The model under review builds one solid part; all positions refer to its coordinate system, in mm. Face numbers are marked on the shaded views. A direction names the side the tool comes from. Give positions to 0.01 mm unless a question says otherwise; leave off trailing zeros. Order: outer loops, then holes, each group sorted by start corner. A loop starts at its lowest first (then second) coordinate and runs counter-clockwise, first axis right, second up. Notation, with made-up numbers: (53, -25) - (89, -25) arc R11 ccw to (89, -16) - close; hole circle Ø3 at (-10, 60.5). An arc over 180 degrees is marked (long way). Put each result on its own line as item: value.
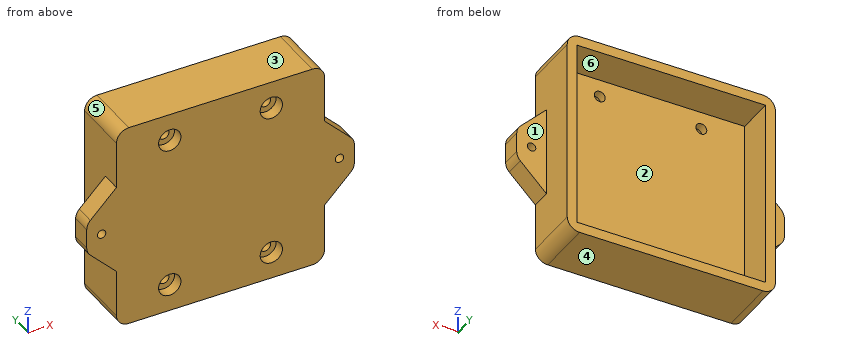
```python
from build123d import *

# Parameters (mm, degrees)
SKETCH1_W           = 84
SKETCH1_H           = 84
SKETCH1_W_2         = 76
SKETCH1_H_2         = 76
SKETCH1_R           = 4.5
SKETCH1_R_2         = 2.2
SKETCH1_W_3         = 12
SKETCH1_H_3         = 12
SKETCH1_R_3         = 1.7
BOSS_EXTRUDE1_DEPTH = 8
SKETCH1_3_W         = 84
SKETCH1_3_H         = 84
SKETCH1_3_W_2       = 76
SKETCH1_3_H_2       = 76
BOSS_EXTRUDE2_DEPTH = 15
SKETCH2_R           = 4.5
CUT_EXTRUDE1_DEPTH  = 4.5
FILLET1_R           = 5


with BuildPart() as part:
    # Sketch1 → Boss-Extrude1 (new body)
    with BuildSketch(Plane(origin=(0, 0, 0), x_dir=(1, 0, 0), z_dir=(0, 1, 0))):
        Rectangle(SKETCH1_W, SKETCH1_H)
        Rectangle(SKETCH1_W_2, SKETCH1_H_2, mode=Mode.SUBTRACT)
        Rectangle(SKETCH1_W_2, SKETCH1_H_2)
        with Locations((20.5, -31)):
            Circle(SKETCH1_R, mode=Mode.SUBTRACT)
        with Locations((-20.5, -31)):
            Circle(SKETCH1_R, mode=Mode.SUBTRACT)
        with Locations((20.5, 31)):
            Circle(SKETCH1_R, mode=Mode.SUBTRACT)
        with Locations((-20.5, 31)):
            Circle(SKETCH1_R, mode=Mode.SUBTRACT)
        with Locations((-20.5, -31)):
            Circle(SKETCH1_R)
        with Locations((-20.5, -31)):
            Circle(SKETCH1_R_2, mode=Mode.SUBTRACT)
        with Locations((-20.5, 31)):
            Circle(SKETCH1_R)
        with Locations((-20.5, 31)):
            Circle(SKETCH1_R_2, mode=Mode.SUBTRACT)
        with Locations((20.5, 31)):
            Circle(SKETCH1_R)
        with Locations((20.5, 31)):
            Circle(SKETCH1_R_2, mode=Mode.SUBTRACT)
        with Locations((20.5, -31)):
            Circle(SKETCH1_R)
        with Locations((20.5, -31)):
            Circle(SKETCH1_R_2, mode=Mode.SUBTRACT)
        Polygon((-42, 6), (-42, 18), (-54, 6), align=None)
        with Locations((-48, 0)):
            Rectangle(SKETCH1_W_3, SKETCH1_H_3)
        with Locations((-48, 0)):
            Circle(SKETCH1_R_3, mode=Mode.SUBTRACT)
        Polygon((-42, -18), (-42, -6), (-54, -6), align=None)
        Polygon((54, 6), (42, 18), (42, 6), align=None)
        with Locations((48, 0)):
            Rectangle(SKETCH1_W_3, SKETCH1_H_3)
        with Locations((48, 0)):
            Circle(SKETCH1_R_3, mode=Mode.SUBTRACT)
        Polygon((54, -6), (42, -6), (42, -18), align=None)
    extrude(amount=-BOSS_EXTRUDE1_DEPTH)

    # Sketch1_3 → Boss-Extrude2 (add)
    with BuildSketch(Plane(origin=(0, 0, 0), x_dir=(1, 0, 0), z_dir=(0, 1, 0))):
        Rectangle(SKETCH1_3_W, SKETCH1_3_H)
        Rectangle(SKETCH1_3_W_2, SKETCH1_3_H_2, mode=Mode.SUBTRACT)
    extrude(amount=BOSS_EXTRUDE2_DEPTH)

    # Sketch2 → Cut-Extrude1 (cut)
    with BuildSketch(Plane.XZ.offset(8)):
        with Locations((-20.5, 31)):
            Circle(SKETCH2_R)
        with Locations((-20.5, -31)):
            Circle(SKETCH2_R)
        with Locations((20.5, -31)):
            Circle(SKETCH2_R)
        with Locations((20.5, 31)):
            Circle(SKETCH2_R)
    extrude(amount=-CUT_EXTRUDE1_DEPTH, mode=Mode.SUBTRACT)

    # Fillet1
    fillet1_edges = [part.edges().sort_by_distance(p)[0] for p in [
        (42, 3.5, 42),
        (-42, 3.5, 42),
        (-54, -4, 6),
        (-54, -4, -6),
        (-42, 3.5, -42),
        (42, 3.5, -42),
        (54, -4, -6),
        (54, -4, 6),
    ]]
    fillet(fillet1_edges, radius=FILLET1_R)


solid = part.part
```
(1) Take a section at C-C, the plane x = -20.5. Write out the cut boundary in (y, z), then the cut area to 3 significant figures.
The answers:
outline: (-8, -42) - (15, -42) - (15, -38) - (0, -38) - (0, -33.2) - (-3.5, -33.2) - (-3.5, -35.5) - (-8, -35.5) - close; (-8, -26.5) - (-3.5, -26.5) - (-3.5, -28.8) - (0, -28.8) - (0, 28.8) - (-3.5, 28.8) - (-3.5, 26.5) - (-8, 26.5) - close; (-8, 35.5) - (-3.5, 35.5) - (-3.5, 33.2) - (0, 33.2) - (0, 38) - (15, 38) - (15, 42) - (-8, 42) - close
area: 680 mm^2
(2) Take a section at D-D, the plane y = 7.25. Write out the cut boundary in (x, z), then the cut area to 3 significant figures.
The answers:
outline: (-42, -37) arc R5 ccw to (-37, -42) - (37, -42) arc R5 ccw to (42, -37) - (42, 37) arc R5 ccw to (37, 42) - (-37, 42) arc R5 ccw to (-42, 37) - close; hole (-38, -38) - (38, -38) - (38, 38) - (-38, 38) - close
area: 1,260 mm^2
(3) Take a section at A-A, the plane x = -48. Write out the cut boundary in (y, z), then the cut area to 3 significant figures.
The answers:
outline: (-8, -12) - (0, -12) - (0, -1.7) - (-8, -1.7) - close; (-8, 1.7) - (0, 1.7) - (0, 12) - (-8, 12) - close
area: 165 mm^2
(4) Clearance check with flat-ended pins moving along their axes: pin 1 Ø2 at (x, z) = (-2.5, -2.5) entering from +Y; pin 2 Ø5.5 at (x, z) = (-20.5, 31) entering from -Y; pin 3 Ø1.5 at (x, y) = (-43, 3) entering from -Z; pin 4 Ø10 at (y, z) = (7.5, -29.5) entering from -X. State where each tip first meets the part, or that it passes through.
The answers:
pin 1: y = 0
pin 2: y = -3.5
pin 3: through
pin 4: x = -42
(5) For the marked faces 5 and 6, list the 3-axis set-ups (+Z, -Z, +X, -X, +Y, -Y) from which the entire face can be reached by the end or side of a thin tool; tool diameter is ignored.
The answers:
face 5: +Z, -X, +Y, -Y
face 6: +Y
(6) The part is to be moulded in two halves that separate along Z. For the marked faces 1, 2, 3 and 4, say which applies: pulls with the +Z half, pulls with the -Z half, needs draft (parallel to the pull), parting line crosses it, or undercut.
The answers:
face 1: needs draft
face 2: undercut
face 3: pulls with the +Z half
face 4: pulls with the -Z half
(7) Take a section at B-B, the plane z = 31. Write out the cut boundary in (x, y), then the cut area to 3 significant figures.
The answers:
outline: (-42, -8) - (-25, -8) - (-25, -3.5) - (-22.7, -3.5) - (-22.7, 0) - (-38, 0) - (-38, 15) - (-42, 15) - close; (-18.3, -3.5) - (-16, -3.5) - (-16, -8) - (16, -8) - (16, -3.5) - (18.3, -3.5) - (18.3, 0) - (-18.3, 0) - close; (22.7, -3.5) - (25, -3.5) - (25, -8) - (42, -8) - (42, 15) - (38, 15) - (38, 0) - (22.7, 0) - close
area: 680 mm^2
(8) Wall thickness on L1, parallel to X at y = -5.25, z = 30.5; L2, parallel to X at y = -1.1, z = 31; L3, parallel to Z at x = 20.5, y = -5.6: over which ranges is each line inside the solid? List them lowest first.
The answers:
L1: -42 to -24.97, -16.03 to 16.03, 24.97 to 42
L2: -42 to -22.7, -18.3 to 18.3, 22.7 to 42
L3: -42 to -35.5, -26.5 to 26.5, 35.5 to 42
